```python
from build123d import *

# Parameters (mm, degrees)
F0_W         = 99.7252352536
F0_H         = 16.7486164719
F1_DEPTH     = 2.54
F2_R         = 5.08
F3_R         = 8.5048235264
F4_DEPTH     = 2.54
F5_W         = 82.7053110433
F5_H         = 2.5119255297
F6_DEPTH     = 2.54
F7_R         = 1.27
F8_T1_DEPTH  = 2.54
F9_R         = 1.27
F10_T1_DEPTH = 2.54
F11_R        = 1.27
F12_R        = 1.27


# Not quite as in the source:
# - a fillet or chamfer that OpenCascade refuses, or shapes differently, is made with other operations: its cross-section is extruded or revolved along the edge and cut away or added


with BuildPart() as f1:
    # F0 (on Top) → F1 (new body)
    with BuildSketch(Plane.XY):
        with Locations((-11.1071113497, -8.3743082359)):
            Rectangle(F0_W, F0_H)
    extrude(amount=F1_DEPTH)

    # F2
    f2_edges = [f1.edges().sort_by_distance(p)[0] for p in [
        (-60.969729, -16.748616, 1.27),
    ]]
    fillet(f2_edges, radius=F2_R)

    # F3 (on face) → F4 (cut)
    with BuildSketch(Plane.XY.offset(2.54)):
        with Locations((38.7555062771, -8.3743082359)):
            Circle(F3_R)
    extrude(amount=-F4_DEPTH, mode=Mode.SUBTRACT)

    # F5 (on face) → F6 (cut)
    with BuildSketch(Plane(origin=(0, 0, 0), x_dir=(1, 0, 0), z_dir=(0, 0, -1))):
        with Locations((-14.5370734549, 7.9348592553)):
            Rectangle(F5_W, F5_H)
    extrude(amount=-F6_DEPTH, mode=Mode.SUBTRACT)

    # F7
    f7_edges = [f1.edges().sort_by_distance(p)[0] for p in [
        (-55.889729, -9.190822, 1.27),
    ]]
    fillet(f7_edges, radius=F7_R)

    # F8: fillet of radius 1.27 on 1 edges, made by hand

    # F8_s2 → F8_t1 (join)
    with BuildSketch(Plane.XY):
        with BuildLine():
            ThreePointArc((-55.8897289765, -7.9488964905), (-55.5177545886, -7.0508708784), (-54.6197289765, -6.6788964905))
            Line((-54.6197289765, -6.6788964905), (-55.8897289765, -6.6788964905))
            Line((-55.8897289765, -6.6788964905), (-55.8897289765, -7.9488964905))
        make_face()
    extrude(amount=F8_T1_DEPTH)

    # F9
    f9_edges = [f1.edges().sort_by_distance(p)[0] for p in [
        (26.815582, -6.678896, 1.27),
    ]]
    fillet(f9_edges, radius=F9_R)

    # F10: fillet of radius 1.27 on 1 edges, made by hand

    # F10_s2 → F10_t1 (join)
    with BuildSketch(Plane.XY):
        with BuildLine():
            ThreePointArc((26.8155820668, -7.9208220202), (26.4436076789, -8.8188476323), (25.5455820668, -9.1908220202))
            Line((25.5455820668, -9.1908220202), (26.8155820668, -9.1908220202))
            Line((26.8155820668, -9.1908220202), (26.8155820668, -7.9208220202))
        make_face()
    extrude(amount=F10_T1_DEPTH)

    # F11
    f11_edges = [f1.edges().sort_by_distance(p)[0] for p in [
        (37.271261, -16.748616, 1.27),
    ]]
    fillet(f11_edges, radius=F11_R)

    # F12
    f12_edges = [f1.edges().sort_by_distance(p)[0] for p in [
        (37.271261, 0, 1.27),
    ]]
    fillet(f12_edges, radius=F12_R)


solid = f1.part
```
Input: part model. Units: mm. Frame: model coordinates. A direction names the side the tool comes from. Give positions to 0.01 mm unless a question says otherwise; leave off trailing zeros. Loops run counter-clockwise (first coordinate to the right, second up) from the corner with the lowest first, then second, coordinate; pieces in that order, holes last.
1) Section query A-A on x = -46. Return the cut outline in (y, z), and give its area (3 significant figures).
A:
outline: (-16.75, 0) - (-9.19, 0) - (-9.19, 2.54) - (-16.75, 2.54) - close; (-6.68, 0) - (0, 0) - (0, 2.54) - (-6.68, 2.54) - close
area: 36.2 mm2
2) Section query C-C on y = -12.75. Return the cut outline in (x, z), and give its area (3 significant figures).
A:
outline: (-60.85, 0) - (31.46, 0) - (31.46, 2.54) - (-60.85, 2.54) - close
area: 234 mm2
3) Section query B-B on z = 1.9. Return the cut outline in (x, y), and give its area (3 significant figures).
A:
outline: (-60.97, -11.67) arc R5.08 ccw to (-55.89, -16.75) - (32.04, -16.75) arc R1.27 ccw to (32.91, -14.56) arc R8.5 cw to (32.91, -2.19) arc R1.27 ccw to (32.04, 0) - (-60.97, 0) - close; hole (-55.89, -7.93) arc R1.27 ccw to (-54.62, -9.19) - (25.55, -9.19) arc R1.27 ccw to (26.82, -7.93) arc R1.27 ccw to (25.55, -6.68) - (-54.62, -6.68) arc R1.27 ccw to start
area: 1,340 mm2
4) Line query: L1, parallel to Y at x = -8, z = 1.3; L2, parallel to X at y = -8, z = 0.85; L3, parallel to X at y = -8.75, z = 1.15. Output: solid intervals per line, ascending.
A:
L1: y = -16.75 to -9.19, -6.68 to 0
L2: x = -60.97 to -55.89, 26.81 to 30.26
L3: x = -60.97 to -55.58, 26.51 to 30.26
5) Mould query, pull axis Y, two halves, no side actions, for faces 1 (the flat face through (-15, 0, 1)), 2 (the flat face through (-15, -6.679, 1)), 3 (the flat face through (-14, -10, 0)). Classes: released by +Y, released by -Y, zero draft, split by the parting line, or undercut.
A:
face 1: released by +Y
face 2: undercut
face 3: zero draft
6) Section query D-D on y = -3.5. Return the cut outline in (x, z).
A:
outline: (-60.97, 0) - (31.79, 0) - (31.79, 2.54) - (-60.97, 2.54) - close
7) Reachability of faces 4 (the cylindrical face through (-59.52, -15.22, 1.29)), 5 (the flat face through (-15, -9.191, 1)) from +Z, -Z, +X, -X, +Y, -Y: full face, straight path, thin tool, end or side. Return the list, or none.
A:
face 4: +Z, -Z, -X, -Y
face 5: +Z, -Z
